from build123d import *

# Parameters (mm, degrees)
F0_R     = 21
F1_DEPTH = 30
F2_W     = 30
F2_H     = 22
F4_R     = 21
F5_DEPTH = 30
F6_SCALE = 0.9
F8_DEPTH = 25


with BuildPart() as f1:
    # F0 (on Right) → F1 (new body)
    with BuildSketch(Plane.YZ):
        Circle(F0_R)
    extrude(amount=F1_DEPTH)

    # F2 (on Top) → F3 (revolve)
    with BuildSketch(Plane.XY):
        with BuildLine():
            ThreePointArc((30, 27), (15.2069063257, 23.2585620455), (0, 22))
            Line((0, 22), (30, 22))
            Line((30, 22), (30, 27))
        make_face()
        with Locations((15, 11)):
            Rectangle(F2_W, F2_H)
    revolve(axis=Axis((15, 0, 0), (1, 0, 0)))

    # F4 (on face) → F5 (cut)
    with BuildSketch(Plane(origin=(0, 0, 0), x_dir=(0, -1, 0), z_dir=(-1, 0, 0))):
        Circle(F4_R)
    extrude(amount=-F5_DEPTH, mode=Mode.SUBTRACT)


with BuildPart() as f6_1:
    # F6: copy of F1
    add(f1.part.scale(F6_SCALE))


with BuildPart() as f1_1:
    add(f1.part)

    # F7: cut F6_1
    add(f6_1.part, mode=Mode.SUBTRACT)

    # F8 (cut): a face of the model
    f8_faces = [f1_1.faces().sort_by_distance(p)[0] for p in [
        (27, -23.6126922087, 0),
    ]]
    extrude(f8_faces, amount=-F8_DEPTH, mode=Mode.SUBTRACT)


solid = f1_1.part
The listing builds one solid part. Answer for the finished solid, in the listing's coordinates (mm). Give positions to 0.01 mm unless a question says otherwise; leave off trailing zeros. Loops run counter-clockwise (first coordinate to the right, second up) from the corner with the lowest first, then second, coordinate; pieces in that order, holes last.
Item 1: A cutting plane is placed at A-A (y = 0). Give the vertices of the cut face in (x, z), then the cut area to 3 significant figures.
Derived:
outline: (0, -22) arc R92.5 cw to (30, -27) - (30, -24.3) - (27, -24.3) arc R83.25 ccw to (14.08, -21) - (0, -21) - close; (0, 21) - (14.08, 21) arc R83.25 ccw to (27, 24.3) - (30, 24.3) - (30, 27) arc R92.5 cw to (0, 22) - close
area: 101 mm2
Item 2: Find the intervals of material crossed by line 1 along Y through (x, z) = (16.5, 17); line 2 along Z through (x, y) = (18.75, 1); line 3 along Z through (x, y) = (28.15, 0), in increasing order.
Derived:
line 1: y = -16.2 to -13.08, 13.08 to 16.2
line 2: z = -23.9 to -21.92, 21.92 to 23.9
line 3: z = -26.39 to -24.3, 24.3 to 26.39
Item 3: Each of these flat-tipped pins is pushed along its axis until it touches: pin 1 Ø1.5 at (x, y) = (16.5, 17.5) entering from +Z; pin 2 Ø3 at (x, z) = (17.5, -7.5) entering from -Y; pin 3 Ø8 at (x, z) = (3.5, -7) entering from -Y. Where does it stop, or does it pass through?
Derived:
pin 1: stops at z = 16.48
pin 2: stops at y = -23
pin 3: stops at y = -21.89
Item 4: A cutting plane is placed at C-C (x = 13.25). Give the vertices of the cut face in (y, z), then the cut area to 3 significant figures.
Derived:
outline: circle Ø45.91 at (0, 0); hole circle Ø42 at (0, 0)
area: 270 mm2
Item 5: Determine the mould class of faces 1 (the flat face through (30, 24.13, 4.13)), 2 (the cylindrical face through (6.94, -20.03, 6.31)) for opening direction Z: +Z half, -Z half, draft (parallel to the pull), parting line (faces both ways), or undercut.
Derived:
face 1: draft
face 2: undercut
